Model file for the job. Use its own axes, mm. A direction names the side the tool comes from. Coordinates: 2 decimals unless noted, no trailing zeros. Order: outer loops, then holes, each group sorted by start corner. A loop starts at its lowest first (then second) coordinate and runs counter-clockwise, first axis right, second up. Notation, with made-up numbers: (49, 61.5) -> (54, 61.5) arc R23 cw to (54, 81.5) -> close; hole circle Ø1 at (33, -22). An arc over 180 degrees is marked (long way). Use CSV: the item, a comma, the result in double quotes. Start each with the question number.
(1) Pull direction Z, two halves, no side cores. Call faces 4 (the conical face through (-0.15, -4.09, 14.37)), 5 (the flat face through (-5, -6, 22)), 6 (the flat face through (0, -3, 13)), 7 (the conical face through (-0.15, -7.87, 14.38)): pulls with the +Z half, pulls with the -Z half, needs draft (parallel to the pull), parting line crosses it, or undercut.
(2) Cut at C-C on x = 0. Write the cut outline in (y, z).
(3) Pin check, flat tips, straight feed: pin 1 Ø3 at (x, y) = (-0.5, 7) entering from +Z; pin 2 Ø1 at (x, y) = (1, -0.5) entering from +Z; pin 3 Ø1 at (x, z) = (0.5, 16) entering from +Y. Stop position of each tip, or through.
(4) Cut at B-B on z = 19.5. Write the cut outline in (x, y), plus the area to 3 significant figures.
(5) Probe L1, parallel to Y at x = 0, z = 10.5; L2, parallel to Y at x = 0, z = 5; L3, parallel to X at y = -6, z = 4.75. List the from-to ranges inside material, lowest first.
(6) Cut at D-D on x = -8.25. Write the cut outline in (y, z).
(7) Cut at A-A on z = 9.5. Write the cut outline in (x, y).
(8) Tool access for faces 1 (the flat face through (-8.5, -6, 14.5)), 2 (the conical face through (-0.15, 5.03, 14.56)), 3 (the flat face through (0, 3, 13)): list every direction of +Z, -Z, +X, -X, +Y, -Y with a clear straight run to the whole face (end or side of a thin tool).
```python
from build123d import *

# Parameters (mm, degrees)
SKETCH1_W               = 20
SKETCH1_H               = 18
BOSS_EXTRUDE1_DEPTH     = 7
SKETCH2_W               = 20
SKETCH2_H               = 6
BOSS_EXTRUDE2_DEPTH     = 15
SKETCH3_R               = 5.35
CUT_EXTRUDE1_DEPTH      = 18
SKETCH5_W               = 14
SKETCH5_H               = 6
CUT_EXTRUDE2_DEPTH      = 3.85
FILLET1_R               = 0.3
SKETCH6_W               = 20
SKETCH6_H               = 9
CUT_EXTRUDE3_DEPTH      = 16.0000001
CUT_EXTRUDE3_DEPTH_BACK = 8
SKETCH7_R               = 1.5
CUT_EXTRUDE4_DEPTH      = 1
CUT_EXTRUDE4_DEPTH_BACK = 23.0000001


with BuildPart() as part:
    # Sketch1 → Boss-Extrude1 (new body)
    with BuildSketch(Plane.XY):
        Rectangle(SKETCH1_W, SKETCH1_H)
    extrude(amount=BOSS_EXTRUDE1_DEPTH)

    # Sketch2 → Boss-Extrude2 (add)
    with BuildSketch(Plane.XY.offset(7)):
        with Locations((0, -6)):
            Rectangle(SKETCH2_W, SKETCH2_H)
        with Locations((0, 6)):
            Rectangle(SKETCH2_W, SKETCH2_H)
    extrude(amount=BOSS_EXTRUDE2_DEPTH)

    # Sketch3 → Cut-Extrude1 (cut)
    with BuildSketch(Plane.XZ.offset(9)):
        with Locations((0, 19.5)):
            Circle(SKETCH3_R)
        Polygon((-7, 22), (-10, 7), (-10, 22), align=None)
        Polygon((7, 22), (10, 22), (10, 7), align=None)
    extrude(amount=-CUT_EXTRUDE1_DEPTH, mode=Mode.SUBTRACT)

    # Sketch4 → Revolve4 (revolve)
    with BuildSketch(Plane.XY.offset(19.5)):
        with BuildLine():
            Line((-5.35, -3), (-5.35, -9))
            Line((-5.35, -9), (-4.781378582, -6.156892908))
            ThreePointArc((-4.781378582, -6.156892908), (-4.765843122, -6), (-4.781378582, -5.843107092))
            Line((-4.781378582, -5.843107092), (-5.35, -3))
        make_face()
    revolve(axis=Axis((0, -3, 19.5), (0, -1, 0)))

    # Sketch5 → Cut-Extrude2 (cut, through all)
    with BuildSketch(Plane.XY.offset(22)):
        with Locations((0, -6)):
            Rectangle(SKETCH5_W, SKETCH5_H)
    extrude(amount=CUT_EXTRUDE2_DEPTH, mode=Mode.SUBTRACT)

    # Fillet1
    fillet1_edges = [part.edges().sort_by_distance(p)[0] for p in [
        (7, -6, 22),
        (-7, -6, 22),
        (-7, 6, 22),
        (7, 6, 22),
        (-4.729957717, 6, 22),
        (4.729957717, 6, 22),
    ]]
    fillet(fillet1_edges, radius=FILLET1_R)

    # Sketch6 → Cut-Extrude3 (cut, two sides)
    with BuildSketch(Plane.XY.offset(7)) as cut_extrude3_sk:
        with Locations((0, 4.5)):
            Rectangle(SKETCH6_W, SKETCH6_H)
    extrude(amount=CUT_EXTRUDE3_DEPTH, mode=Mode.SUBTRACT)
    extrude(cut_extrude3_sk.sketch, amount=-CUT_EXTRUDE3_DEPTH_BACK, mode=Mode.SUBTRACT)

    # Mirror2: part across plane


with BuildPart() as part_1:
    add(part.part)
    add(part.part.mirror(Plane(origin=(-10, 0, 0), x_dir=(0, 0, 1), z_dir=(0, -1, 0))))

    # Sketch7 → Cut-Extrude4 (cut, two sides)
    with BuildSketch(Plane(origin=(0, 0, 0), x_dir=(-1, 0, 0), z_dir=(0, 0, -1))) as cut_extrude4_sk:
        with Locations((0, -6)):
            Circle(SKETCH7_R)
    extrude(amount=CUT_EXTRUDE4_DEPTH, mode=Mode.SUBTRACT)
    extrude(cut_extrude4_sk.sketch, amount=-CUT_EXTRUDE4_DEPTH_BACK, mode=Mode.SUBTRACT)


solid = part_1.part
```
Outcome:
1,face 4,"undercut"
1,face 5,"pulls with the +Z half"
1,face 6,"needs draft"
1,face 7,"undercut"
2,outline,"(-9, 0) -> (-7.5, 0) -> (-7.5, 14.45) -> (-9, 14.15) -> close; (-4.5, 0) -> (9, 0) -> (9, 14.15) -> (6.16, 14.72) arc R0.8 ccw to (5.84, 14.72) -> (3, 14.15) -> (3, 7) -> (-3, 7) -> (-3, 14.15) -> (-4.5, 14.45) -> close"
3,pin 1,"z = 15.05"
3,pin 2,"z = 7"
3,pin 3,"through"
4,outline,"(-7.5, -9) -> (-5.35, -9) -> (-4.78, -6.16) arc R0.8 ccw to (-4.78, -5.84) -> (-5.35, -3) -> (-7.5, -3) -> close; (-7.5, 3) -> (-5.35, 3) -> (-4.78, 5.84) arc R0.8 ccw to (-4.78, 6.16) -> (-5.35, 9) -> (-7.5, 9) -> close; (4.78, -6.16) -> (5.35, -9) -> (7.5, -9) -> (7.5, -3) -> (5.35, -3) -> (4.78, -5.84) arc R0.8 ccw to start; (4.78, 5.84) -> (5.35, 3) -> (7.5, 3) -> (7.5, 9) -> (5.35, 9) -> (4.78, 6.16) arc R0.8 ccw to start"
4,area,"58.8 mm2"
5,L1,"-9 to -7.5, -4.5 to -3, 3 to 9"
5,L2,"-9 to -7.5, -4.5 to 9"
5,L3,"-10 to -1.5, 1.5 to 10"
6,outline,"(-9, 0) -> (9, 0) -> (9, 15.75) -> (3, 15.75) -> (3, 7) -> (-3, 7) -> (-3, 15.75) -> (-9, 15.75) -> close"
7,outline,"(-9.5, -9) -> (9.5, -9) -> (9.5, -3) -> (-9.5, -3) -> close; (-9.5, 3) -> (9.5, 3) -> (9.5, 9) -> (-9.5, 9) -> close; hole circle Ø3 at (0, -6)"
8,face 1,"+Z, -X, +Y, -Y"
8,face 2,"none"
8,face 3,"+Z, +X, -X"
